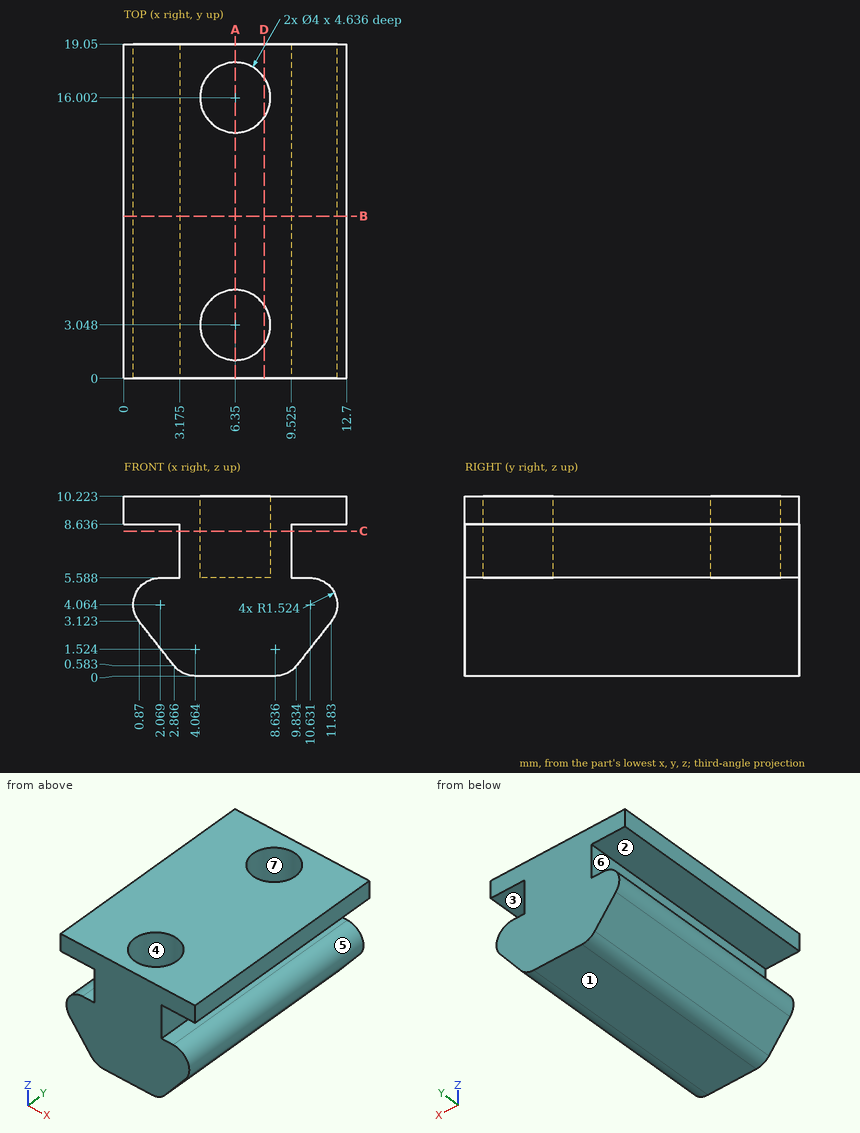
For this review, use the dimensioned drawing (mm, ordinates from the lowest corner) and the shaded views. A direction names the side the tool comes from. Give positions to 0.01 mm unless a question says otherwise; leave off trailing zeros. Write each loop counter-clockwise with the first axis right and the second up, starting at its lowest first coordinate (ties: lowest second). Pieces come first, ordered by that corner, then holes.
(1) Consider section A-A, the plane x = 6.35. Give the boundary of the cut face in (y, z), and give its area (3 significant figures).
(2) Consider section C-C, the plane z = 8.25. Give the number of separate pieces and of enclosed holes in the cut face.
(3) To check wall thickness, follow L1, parallel to Y at x = 6.35, z = 8.9; L2, parallel to Z at x = 2, y = 4.5 (1 decimal); L3, parallel to Z at x = 11.75, y = 1.5 (1 decimal). State the ranges of each line that lie inside material, in increasing order.
(4) Consider section B-B, the plane y = 9.25. Give the boundary of the cut face in (x, z) (1 decimal).
(5) Consider section D-D, the plane x = 8. Give the boundary of the cut face in (y, z), and give its area (3 significant figures).
(6) Tool access review of the marked faces 1, 2, 3 and 4: name each direction out of +Z, -Z, +X, -X, +Y, -Y from which nothing blocks a thin tool from reaching the whole face with its end or side.
(7) The part is to be moulded in two halves that separate along X. For the marked faces 5, 6 and 7, say which applies: released by +X, released by -X, zero draft, split by the parting line, or undercut.
(8) For P1, Ø2, axis at x = 2.5, y = 7, coming from the -Z side; P2, Ø1.6, axis at x = 2, y = 5.5, coming from the -Z side (1 decimal); P3, Ø1, axis at x = 10.5, y = 13.5, coming from the -Z side (1 decimal), all flat-tipped, find the tip position at first contact; note any pin that passes through.
Returned:
1. outline: (0, 0) - (19.05, 0) - (19.05, 10.22) - (18, 10.22) - (18, 5.59) - (14, 5.59) - (14, 10.22) - (5.05, 10.22) - (5.05, 5.59) - (1.05, 5.59) - (1.05, 10.22) - (0, 10.22) - close
1. area: 158 mm2
2. separate pieces: 1
2. enclosed holes: 2
3. L1: y = 0 to 1.05, 5.05 to 14, 18 to 19.05
3. L2: z = 1.7 to 5.6, 8.6 to 10.2
3. L3: z = 3 to 5.1, 8.6 to 10.2
4. outline: (0, 8.6) - (3.2, 8.6) - (3.2, 5.6) - (2.1, 5.6) arc R1.5 ccw to (0.9, 3.1) - (2.9, 0.6) arc R1.5 ccw to (4.1, 0) - (8.6, 0) arc R1.5 ccw to (9.8, 0.6) - (11.8, 3.1) arc R1.5 ccw to (10.6, 5.6) - (9.5, 5.6) - (9.5, 8.6) - (12.7, 8.6) - (12.7, 10.2) - (0, 10.2) - close
5. outline: (0, 0) - (19.05, 0) - (19.05, 10.22) - (17.13, 10.22) - (17.13, 5.59) - (14.87, 5.59) - (14.87, 10.22) - (4.18, 10.22) - (4.18, 5.59) - (1.92, 5.59) - (1.92, 10.22) - (0, 10.22) - close
5. area: 174 mm2
6. face 1: -Z, +X, -X, +Y, -Y
6. face 2: -X, +Y, -Y
6. face 3: +X, +Y, -Y
6. face 4: +Z
7. face 5: released by +X
7. face 6: released by -X
7. face 7: undercut
8. P1: stops at z = 0.11
8. P2: stops at z = 0.7
8. P3: stops at z = 0.8
